from build123d import *

# Parameters (mm, degrees)
SKETCH_1_R          = 9.5
SKETCH_1_R_2        = 5
EXTRUDE_1_DEPTH     = 5
SKETCH_2_R          = 8.25
SKETCH_2_R_2        = 6.25
CUT_EXTRUDE_1_DEPTH = 0.2
SKETCH_3_R          = 8.75
SKETCH_3_R_2        = 6.25
CUT_EXTRUDE_2_DEPTH = 0.2
CHAMFER_2_SIZE      = 0.1


with BuildPart() as part:
    # 草图1 → 凸台-拉伸1 (new body)
    with BuildSketch(Plane(origin=(0, 0, 0), x_dir=(0, 0, -1), z_dir=(1, 0, 0))):
        Circle(SKETCH_1_R)
        Circle(SKETCH_1_R_2, mode=Mode.SUBTRACT)
    extrude(amount=EXTRUDE_1_DEPTH)

    # 草图2 → 切除-拉伸1 (cut)
    with BuildSketch(Plane.ZY):
        with Locations((0.111641095, 0)):
            Circle(SKETCH_2_R)
        with Locations((0.111641095, 0)):
            Circle(SKETCH_2_R_2, mode=Mode.SUBTRACT)
    extrude(amount=-CUT_EXTRUDE_1_DEPTH, mode=Mode.SUBTRACT)

    # 草图3 → 切除-拉伸2 (cut)
    with BuildSketch(Plane(origin=(5, 0, 0), x_dir=(0, 0, -1), z_dir=(1, 0, 0))):
        Circle(SKETCH_3_R)
        Circle(SKETCH_3_R_2, mode=Mode.SUBTRACT)
    extrude(amount=-CUT_EXTRUDE_2_DEPTH, mode=Mode.SUBTRACT)

    # 倒角2
    chamfer_2_edges = [part.edges().sort_by_distance(p)[0] for p in [
        (0, 0, 5),
        (5, 0, 5),
    ]]
    chamfer(chamfer_2_edges, length=CHAMFER_2_SIZE)


solid = part.part
Work out the finished part from the listing and answer in its coordinate system (mm). A direction names the side the tool comes from. Round coordinates to 2 decimals unless told otherwise and drop trailing zeros. Order: outer loops, then holes, each group sorted by start corner. A loop starts at its lowest first (then second) coordinate and runs counter-clockwise, first axis right, second up. Notation, with made-up numbers: M -23.75,63 L 14.25,63 A17 cw 14.25,88 Z; hole C 10.25,62.25 d11. An arc over 180 degrees is marked long. Put each result on its own line as item: value. Start each with the question number.
Q1. Straight lines are drawn through the part: L1, parallel to X at y = 3.75, z = -7.5; L2, parallel to Z at x = 2.2, y = -0.5; L3, parallel to X at y = 7.25, z = -3.75. For each, find the intervals that lie inside material, in ascending order. Write a range as [from, to].
Q2. Section D-D, the plane z = -7.5 is taken. Write down the section's boundary in (x, y).
Q3. Section A-A, the plane y = 0 is taken. Write down the section's boundary in (x, z).
Q4. A tool of negligible diameter and unlimited length cuts with its end or side. For faces 5 (the flat face through (0, 8, -3)), 6 (the flat face through (4.8, -6, -4)), from which of +Z, -Z, +X, -X, +Y, -Y can it reach the whole face along a straight path? Write none if from no direction.
Q5. Section B-B, the plane z = 0 is taken. Write down the section's boundary in (x, y), and give its area (3 significant figures).
Q6. For a pull along Y with two mould halves and no side action, classify faces 1 (the flat face through (0, -2, 5)), 2 (the flat face through (0.2, 6, 3)), 3 (the cylindrical face through (2.47, -4.88, 1.08)), 4 (the cylindrical face through (2.46, -8.43, -4.38)) as pulls with the +Y half, pulls with the -Y half, needs draft (parallel to the pull), parting line crosses it, or undercut.
Q7. Flat-ended cylindrical pins translate along their axes: pin 1 (10.5 mm diameter, centred on y = 0, z = 0, fed in from +X); pin 2 (3 mm diameter, centred on x = 4.5, y = 2.5, fed in from +Z); pin 3 (1 mm diameter, centred on x = 4.5, y = 4, fed in from -Z); pin 4 (3 mm diameter, centred on x = 0.5, z = 4, fed in from -Y). Find the tip coordinate at first contact, or state that the pin passes through.
Q8. Section C-C, the plane x = 4.15 is taken. Write down the section's boundary in (y, z).
Findings below:
1. L1: x = [0, 4.8]
1. L2: z = [-9.49, -4.97], [4.97, 9.49]
1. L3: x = [0.2, 4.8]
2. outline: M 0,-5.83 L 5,-5.83 L 5,-4.51 L 4.8,-4.51 L 4.8,4.51 L 5,4.51 L 5,5.83 L 0,5.83 L 0,3.18 L 0.2,3.18 L 0.2,-3.18 L 0,-3.18 Z
3. outline: M 0,-9.5 L 5,-9.5 L 5,-8.75 L 4.8,-8.75 L 4.8,-6.25 L 5,-6.25 L 5,-5.1 L 4.9,-5 L 0.1,-5 L 0,-5.1 L 0,-6.14 L 0.2,-6.14 L 0.2,-8.14 L 0,-8.14 Z; M 0,5.1 L 0.1,5 L 4.9,5 L 5,5.1 L 5,6.25 L 4.8,6.25 L 4.8,8.75 L 5,8.75 L 5,9.5 L 0,9.5 L 0,8.36 L 0.2,8.36 L 0.2,6.36 L 0,6.36 Z
4. face 5: +Z, -Z, -X, +Y, -Y
4. face 6: +X
5. outline: M 0,-9.5 L 5,-9.5 L 5,-8.75 L 4.8,-8.75 L 4.8,-6.25 L 5,-6.25 L 5,-5.1 L 4.9,-5 L 0.1,-5 L 0,-5.1 L 0,-6.25 L 0.2,-6.25 L 0.2,-8.25 L 0,-8.25 Z; M 0,5.1 L 0.1,5 L 4.9,5 L 5,5.1 L 5,6.25 L 4.8,6.25 L 4.8,8.75 L 5,8.75 L 5,9.5 L 0,9.5 L 0,8.25 L 0.2,8.25 L 0.2,6.25 L 0,6.25 Z
5. area: 43.2 mm^2
6. face 1: needs draft
6. face 2: undercut
6. face 3: undercut
6. face 4: parting line crosses it
7. pin 1: stops at x = 5
7. pin 2: stops at z = 9.45
7. pin 3: stops at z = -8.83
7. pin 4: stops at y = -9.17
8. outline: C 0,0 d19; hole C 0,0 d10
